from build123d import *

# Parameters (mm, degrees)
SKETCH1_R                     = 11
BOSS_EXTRUDE1_DEPTH           = 2
SKETCH2_R                     = 7
BOSS_EXTRUDE2_DEPTH           = 2.2
SKETCH3_R                     = 5.5
BOSS_EXTRUDE3_DEPTH           = 1
BOSS_EXTRUDE4_DEPTH           = 0.4
BOSS_EXTRUDE5_DEPTH           = 3
SKETCH6_W                     = 1.66
SKETCH6_H                     = 0.4
BOSS_EXTRUDE6_DEPTH           = 2
BOSS_EXTRUDE6_DRAFT           = 2
SKETCH6_W_2                   = 1.289820998
BOSS_EXTRUDE6_PROFILE_2_DEPTH = 2
BOSS_EXTRUDE6_PROFILE_2_DRAFT = 2
BOSS_EXTRUDE6_PROFILE_3_DEPTH = 2
BOSS_EXTRUDE6_PROFILE_3_DRAFT = 2
BOSS_EXTRUDE6_PROFILE_4_DEPTH = 2
BOSS_EXTRUDE6_PROFILE_4_DRAFT = 2
BOSS_EXTRUDE6_PROFILE_5_DEPTH = 2
BOSS_EXTRUDE6_PROFILE_5_DRAFT = 2
SKETCH7_W                     = 17.2
SKETCH7_H                     = 6.6
CUT_EXTRUDE1_DEPTH            = 2


with BuildPart() as part:
    # Sketch1 → Boss-Extrude1 (new body)
    with BuildSketch(Plane.XY):
        Circle(SKETCH1_R)
    extrude(amount=BOSS_EXTRUDE1_DEPTH)

    # Sketch2 → Boss-Extrude2 (add)
    with BuildSketch(Plane(origin=(0, 0, 0), x_dir=(-1, 0, 0), z_dir=(0, 0, -1))):
        with Locations(Location((0, 0, 0), (0, 0, 180))):
            Circle(SKETCH2_R)
    extrude(amount=BOSS_EXTRUDE2_DEPTH)

    # Sketch3 → Boss-Extrude3 (add)
    with BuildSketch(Plane(origin=(0, 0, -2.2), x_dir=(-1, 0, 0), z_dir=(0, 0, -1))):
        Circle(SKETCH3_R)
    extrude(amount=BOSS_EXTRUDE3_DEPTH)

    # Sketch4 → Boss-Extrude4 (add)
    with BuildSketch(Plane(origin=(0, 0, -3.2), x_dir=(-1, 0, 0), z_dir=(0, 0, -1))):
        Polygon((-4, 3.774917218), (4, 3.774917218), (8.6, -5), (8.6, -18), (7.6, -18), (6.9, -11), (5.1, -11), (5.1, -2.059126028), (3.85, -2.059126028), (3.5, -18), (2.5, -18), (2.15, -2.059126028), (0.85, -2.059126028), (0.5, -18), (-0.5, -18), (-0.85, -2.059126028), (-2.15, -2.059126028), (-2.5, -18), (-3.5, -18), (-3.85, -2.059126028), (-5.1, -2.059126028), (-5.1, -11), (-6.9, -11), (-7.6, -18), (-8.6, -18), (-8.6, -5), align=None)
    extrude(amount=BOSS_EXTRUDE4_DEPTH)

    # Sketch5 → Boss-Extrude5 (add)
    with BuildSketch(Plane(origin=(0, 0, -3.6), x_dir=(-1, 0, 0), z_dir=(0, 0, -1))):
        Polygon((-8.6, -5), (-4, 3.774917218), (4, 3.774917218), (8.6, -5), align=None)
    extrude(amount=BOSS_EXTRUDE5_DEPTH)


with BuildPart() as boss_extrude6_tool:
    # Sketch6 → Boss-Extrude6 (with draft: the straight prism first)
    with BuildSketch(Plane(origin=(0, 0, -3.6), x_dir=(-1, 0, 0), z_dir=(0, 0, -1))):
        with Locations((7.77, -11.2)):
            Rectangle(SKETCH6_W, SKETCH6_H)
    extrude(amount=BOSS_EXTRUDE6_DEPTH)
    # Boss-Extrude6: the draft: its side faces are tilted about the plane it starts from
    boss_extrude6_sides = [boss_extrude6_tool.faces().sort_by_distance(p)[0] for p in [
        (-8.6, -11.2, -4.6),
        (-7.77, -11, -4.6),
        (-6.94, -11.2, -4.6),
        (-7.77, -11.4, -4.6),
    ]]
    draft(boss_extrude6_sides, Plane(origin=(0, 0, -3.6), x_dir=(-1, 0, 0), z_dir=(0, 0, -1)), BOSS_EXTRUDE6_DRAFT)


with BuildPart() as part_1:
    add(part.part)

    # Boss-Extrude6: add boss_extrude6_tool
    add(boss_extrude6_tool.part)


with BuildPart() as boss_extrude6_profile_2_tool:
    # Sketch6 → Boss-Extrude6 profile 2 (with draft: the straight prism first)
    with BuildSketch(Plane(origin=(0, 0, -3.6), x_dir=(-1, 0, 0), z_dir=(0, 0, -1))):
        with Locations((3, -11.2)):
            Rectangle(SKETCH6_W_2, SKETCH6_H)
    extrude(amount=BOSS_EXTRUDE6_PROFILE_2_DEPTH)
    # Boss-Extrude6 profile 2: the draft: its side faces are tilted about the plane it starts from
    boss_extrude6_profile_2_sides = [boss_extrude6_profile_2_tool.faces().sort_by_distance(p)[0] for p in [
        (-2.355089501, -11.2, -4.6),
        (-3, -11.4, -4.6),
        (-3.644910499, -11.2, -4.6),
        (-3, -11, -4.6),
    ]]
    draft(boss_extrude6_profile_2_sides, Plane(origin=(0, 0, -3.6), x_dir=(-1, 0, 0), z_dir=(0, 0, -1)), BOSS_EXTRUDE6_PROFILE_2_DRAFT)


with BuildPart() as part_2:
    add(part_1.part)

    # Boss-Extrude6 profile 2: add boss_extrude6_profile_2_tool
    add(boss_extrude6_profile_2_tool.part)


with BuildPart() as boss_extrude6_profile_3_tool:
    # Sketch6 → Boss-Extrude6 profile 3 (with draft: the straight prism first)
    with BuildSketch(Plane(origin=(0, 0, -3.6), x_dir=(-1, 0, 0), z_dir=(0, 0, -1))):
        with Locations((0, -11.2)):
            Rectangle(SKETCH6_W_2, SKETCH6_H)
    extrude(amount=BOSS_EXTRUDE6_PROFILE_3_DEPTH)
    # Boss-Extrude6 profile 3: the draft: its side faces are tilted about the plane it starts from
    boss_extrude6_profile_3_sides = [boss_extrude6_profile_3_tool.faces().sort_by_distance(p)[0] for p in [
        (0.644910499, -11.2, -4.6),
        (0, -11.4, -4.6),
        (-0.644910499, -11.2, -4.6),
        (0, -11, -4.6),
    ]]
    draft(boss_extrude6_profile_3_sides, Plane(origin=(0, 0, -3.6), x_dir=(-1, 0, 0), z_dir=(0, 0, -1)), BOSS_EXTRUDE6_PROFILE_3_DRAFT)


with BuildPart() as part_3:
    add(part_2.part)

    # Boss-Extrude6 profile 3: add boss_extrude6_profile_3_tool
    add(boss_extrude6_profile_3_tool.part)


with BuildPart() as boss_extrude6_profile_4_tool:
    # Sketch6 → Boss-Extrude6 profile 4 (with draft: the straight prism first)
    with BuildSketch(Plane(origin=(0, 0, -3.6), x_dir=(-1, 0, 0), z_dir=(0, 0, -1))):
        with Locations((-3, -11.2)):
            Rectangle(SKETCH6_W_2, SKETCH6_H)
    extrude(amount=BOSS_EXTRUDE6_PROFILE_4_DEPTH)
    # Boss-Extrude6 profile 4: the draft: its side faces are tilted about the plane it starts from
    boss_extrude6_profile_4_sides = [boss_extrude6_profile_4_tool.faces().sort_by_distance(p)[0] for p in [
        (3.644910499, -11.2, -4.6),
        (3, -11.4, -4.6),
        (2.355089501, -11.2, -4.6),
        (3, -11, -4.6),
    ]]
    draft(boss_extrude6_profile_4_sides, Plane(origin=(0, 0, -3.6), x_dir=(-1, 0, 0), z_dir=(0, 0, -1)), BOSS_EXTRUDE6_PROFILE_4_DRAFT)


with BuildPart() as part_4:
    add(part_3.part)

    # Boss-Extrude6 profile 4: add boss_extrude6_profile_4_tool
    add(boss_extrude6_profile_4_tool.part)


with BuildPart() as boss_extrude6_profile_5_tool:
    # Sketch6 → Boss-Extrude6 profile 5 (with draft: the straight prism first)
    with BuildSketch(Plane(origin=(0, 0, -3.6), x_dir=(-1, 0, 0), z_dir=(0, 0, -1))):
        with Locations((-7.77, -11.2)):
            Rectangle(SKETCH6_W, SKETCH6_H)
    extrude(amount=BOSS_EXTRUDE6_PROFILE_5_DEPTH)
    # Boss-Extrude6 profile 5: the draft: its side faces are tilted about the plane it starts from
    boss_extrude6_profile_5_sides = [boss_extrude6_profile_5_tool.faces().sort_by_distance(p)[0] for p in [
        (6.94, -11.2, -4.6),
        (7.77, -11, -4.6),
        (8.6, -11.2, -4.6),
        (7.77, -11.4, -4.6),
    ]]
    draft(boss_extrude6_profile_5_sides, Plane(origin=(0, 0, -3.6), x_dir=(-1, 0, 0), z_dir=(0, 0, -1)), BOSS_EXTRUDE6_PROFILE_5_DRAFT)


with BuildPart() as part_5:
    add(part_4.part)

    # Boss-Extrude6 profile 5: add boss_extrude6_profile_5_tool
    add(boss_extrude6_profile_5_tool.part)

    # Sketch7 → Cut-Extrude1 (cut)
    with BuildSketch(Plane(origin=(0, 0, -3.6), x_dir=(-1, 0, 0), z_dir=(0, 0, -1))):
        with Locations((0, -14.7)):
            Rectangle(SKETCH7_W, SKETCH7_H)
    extrude(amount=-CUT_EXTRUDE1_DEPTH, mode=Mode.SUBTRACT)


solid = part_5.part
Verification items for the finished model (mm, model axes). A direction names the side the tool comes from. Coordinates: 2 decimals unless noted, no trailing zeros. Order: outer loops, then holes, each group sorted by start corner. A loop starts at its lowest first (then second) coordinate and runs counter-clockwise, first axis right, second up.
Item 1: Depth check by flat-ended pin: pin 1 (3 mm diameter, centred on y = -6.5, z = 1, fed in from -X); pin 2 (3 mm diameter, centred on y = 2.5, z = -4.5, fed in from +X); pin 3 (1.3 mm diameter, centred on x = 3.5, y = -7.5, fed in from -Z). Enter the tip coordinate at first touch or a pass-through.
Filled in:
pin 1: stops at x = -9.8
pin 2: stops at x = 5.45
pin 3: stops at z = -3.6
Item 2: Section check D-D, the plane y = -10. Enter the section's corners in (x, z).
Filled in:
outline: (-8.6, -3.6) - (-5.1, -3.6) - (-5.1, -3.2) - (-8.6, -3.2) - close; (-4.58, 0) - (4.58, 0) - (4.58, 2) - (-4.58, 2) - close; (-3.68, -3.6) - (-2.32, -3.6) - (-2.32, -3.2) - (-3.68, -3.2) - close; (-0.68, -3.6) - (0.68, -3.6) - (0.68, -3.2) - (-0.68, -3.2) - close; (2.32, -3.6) - (3.68, -3.6) - (3.68, -3.2) - (2.32, -3.2) - close; (5.1, -3.6) - (8.6, -3.6) - (8.6, -3.2) - (5.1, -3.2) - close
Item 3: Section check A-A, the plane z = -5. Enter the section's corners in (x, y), then the cut area to 3 significant figures.
Filled in:
outline: (-8.6, -5) - (8.6, -5) - (4, 3.77) - (-4, 3.77) - close; (-8.55, -11.35) - (-6.99, -11.35) - (-6.99, -11.05) - (-8.55, -11.05) - close; (-3.6, -11.35) - (-2.4, -11.35) - (-2.4, -11.05) - (-3.6, -11.05) - close; (-0.6, -11.35) - (0.6, -11.35) - (0.6, -11.05) - (-0.6, -11.05) - close; (2.4, -11.35) - (3.6, -11.35) - (3.6, -11.05) - (2.4, -11.05) - close; (6.99, -11.35) - (8.55, -11.35) - (8.55, -11.05) - (6.99, -11.05) - close
area: 113 mm2
Item 4: Section check C-C, the plane x = 0. Enter the section's corners in (y, z).
Filled in:
outline: (-11.4, -3.6) - (-11.33, -5.6) - (-11.07, -5.6) - (-11, -3.6) - (-5, -3.6) - (-5, -6.6) - (3.77, -6.6) - (3.77, -3.2) - (5.5, -3.2) - (5.5, -2.2) - (7, -2.2) - (7, 0) - (11, 0) - (11, 2) - (-11, 2) - (-11, 0) - (-7, 0) - (-7, -2.2) - (-5.5, -2.2) - (-5.5, -3.2) - (-11.4, -3.2) - close
Item 5: Access from +Z, -Z, +X, -X, +Y, -Y to the whole of each face (thin tool, end or side, straight path). Record for faces 1 (the face through (3, -8, -3.2)), 2 (the face through (1.19, -5.37, -2.69)), 3 (the face through (0, -5, -5)), 4 (the face through (0, -8, -3.2)), 5 (the face through (1, -4, -3.6)).
Filled in:
face 1: +X, -Y
face 2: none
face 3: -Z, +X, -X
face 4: +X, -X, -Y
face 5: -Y
Item 6: Release check for a two-part mould opening along Z. For faces 6 (the face through (-6.268, -0.551, -4.876)), 7 (the face through (7, -8, -3.6)), 8 (the face through (7, -6, -3.2)) record: +Z half, -Z half, draft (parallel to the pull), parting line (faces both ways), or undercut.
Filled in:
face 6: draft
face 7: -Z half
face 8: undercut
Item 7: Section check B-B, the plane x = -7.75. Enter the section's corners in (y, z), then the cut area to 3 significant figures.
Filled in:
outline: (-11.4, -3.6) - (-11.33, -5.6) - (-11.07, -5.6) - (-11, -3.6) - (-5, -3.6) - (-5, -6.6) - (-3.38, -6.6) - (-3.38, -3.2) - (-11.4, -3.2) - close; (-7.81, 0) - (7.81, 0) - (7.81, 2) - (-7.81, 2) - close
area: 40.0 mm2
Item 8: Material ranges on L1, parallel to Z at x = 5.5, y = -9; L2, parallel to Z at x = 5.25, y = -2.5; L3, parallel to Z at x = 1, y = -7, recorded low to high.
Filled in:
L1: z = -3.6 to -3.2, 0 to 2
L2: z = -6.6 to -3.2, -2.2 to 2
L3: z = 0 to 2
